For this review, take the finished solid that the model builds, in its own axes (mm). Face numbers are marked on the shaded views. A direction names the side the tool comes from. Round coordinates to 2 decimals unless told otherwise and drop trailing zeros. Order: outer loops, then holes, each group sorted by start corner. A loop starts at its lowest first (then second) coordinate and runs counter-clockwise, first axis right, second up. Notation, with made-up numbers: (23.5, -16) -> (46.5, -16) arc R11 ccw to (46.5, 2) -> close; hole circle Ø10 at (-2.75, -21). An arc over 180 degrees is marked (long way). Put each result on its own line as item: value. Start each with the question number.
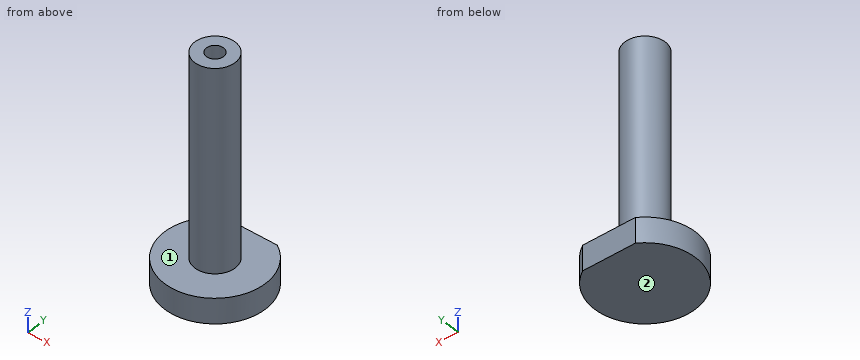
```python
from build123d import *

# Parameters (mm, degrees)
ESQUISSE1_R             = 20
BOSS_EXTRU_1_DEPTH      = 10
ESQUISSE2_R             = 8
BOSS_EXTRU_2_DEPTH      = 80
ESQUISSE3_W             = 36.346174344
ESQUISSE3_H             = 6
ENL_V_MAT_EXTRU_3_DEPTH = 41


with BuildPart() as part:
    # Esquisse1 → Boss.-Extru.1 (new body)
    with BuildSketch(Plane.XY):
        Circle(ESQUISSE1_R)
    extrude(amount=BOSS_EXTRU_1_DEPTH)

    # Esquisse2 → Boss.-Extru.2 (add)
    with BuildSketch(Plane.XY.offset(10)):
        Circle(ESQUISSE2_R)
    extrude(amount=BOSS_EXTRU_2_DEPTH)

    # Esquisse3 → Enlèv. mat.-Extru.3 (cut)
    with BuildSketch(Plane.XY):
        with Locations((0, 20)):
            Rectangle(ESQUISSE3_W, ESQUISSE3_H)
    extrude(amount=ENL_V_MAT_EXTRU_3_DEPTH, mode=Mode.SUBTRACT)

    # Esquisse5 → Trou taraudé M81 (revolve, cut)
    with BuildSketch(Plane(origin=(0, 0, 90), x_dir=(0, -1, 0), z_dir=(1, 0, 0))):
        Polygon((0, 0), (0, 24.292926105), (3.4, 22.25), (3.4, 0), align=None)
    revolve(axis=Axis((0, 0, 96.35), (0, 0, -1)), mode=Mode.SUBTRACT)


solid = part.part
```
Item 1: Tool access review of the marked faces 1 and 2: name each direction out of +Z, -Z, +X, -X, +Y, -Y from which nothing blocks a thin tool from reaching the whole face with its end or side.
Item 2: Consider section A-A, the plane z = 74. Write out the cut boundary in (x, y).
Item 3: Consider section D-D, the plane x = 12.5. Write out the cut boundary in (y, z).
Item 4: Consider section B-B, the plane y = -6. Write out the cut boundary in (x, z), plus the area to 3 significant figures.
Item 5: For L1, parallel to Y at x = 0, z = 73.75; L2, parallel to Z at x = -10, y = -15; L3, parallel to Y at x = -1.5, z = 68, list the stretches that pass through material, from the lowest coordinate up.
Item 6: Consider section C-C, the plane z = 12.5. Write out the cut boundary in (x, y).
Item 7: Insertion check: pin 1 Ø2 at (y, z) = (-1, 76) entering from +X; pin 2 Ø3 at (x, y) = (-2.5, -13.5) entering from -Z; pin 3 Ø6 at (y, z) = (7.5, 44) entering from -X; pin 4 Ø8 at (x, y) = (-7.5, 12.5) entering from +Z. Each pin has a flat end and moves straight along its axis. Give the tip position at first contact, or say it passes through.
Evaluation:
1. face 1: +Z
1. face 2: -Z, +X, -X, +Y, -Y
2. outline: circle Ø16 at (0, 0); hole circle Ø6.8 at (0, 0)
3. outline: (-15.61, 0) -> (15.61, 0) -> (15.61, 10) -> (-15.61, 10) -> close
4. outline: (-19.08, 0) -> (19.08, 0) -> (19.08, 10) -> (5.29, 10) -> (5.29, 90) -> (-5.29, 90) -> (-5.29, 10) -> (-19.08, 10) -> close
4. area: 1,230 mm^2
5. L1: y = -8 to -3.4, 3.4 to 8
5. L2: z = 0 to 10
5. L3: y = -7.86 to -3.05, 3.05 to 7.86
6. outline: circle Ø16 at (0, 0)
7. pin 1: stops at x = 8
7. pin 2: stops at z = 0
7. pin 3: stops at x = -6.61
7. pin 4: stops at z = 10
